Answer from the drawing. Dimensions are ordinates in mm from the lowest x, y and z of the part. Coordinates: 2 decimals unless noted, no trailing zeros. Order: outer loops, then holes, each group sorted by start corner. A loop starts at its lowest first (then second) coordinate and runs counter-clockwise, first axis right, second up.
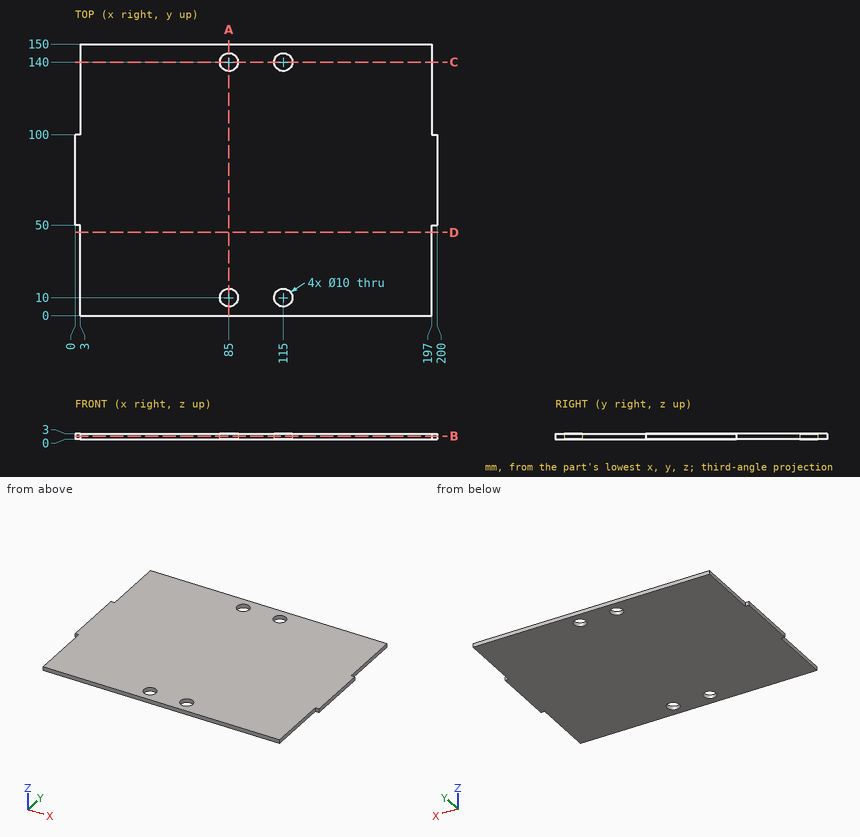
1. The part is cut by section B-B (z = 1.6). Determine the outline of the cut face in (x, y), plus the area to 3 significant figures.
2. Consider probe 1 along Y at (x, z) = (85, 1.95); probe 2 along Y at (x, z) = (84, 2.1); probe 3 along X at (y, z) = (144.5, 0.7). Determine where each line is inside the solid, lowest interval first.
3. The part is cut by section C-C (y = 140). Determine the outline of the cut face in (x, z).
4. The part is cut by section D-D (y = 46). Determine the outline of the cut face in (x, z), plus the area to 3 significant figures.
5. Flat-ended cylindrical pins translate along their axes: pin 1 (1.5 mm diameter, centred on x = 198, z = 1.5, fed in from +Y); pin 2 (1.5 mm diameter, centred on y = 107, z = 0.5, fed in from -X); pin 3 (1.5 mm diameter, centred on x = 1.5, z = 1.5, fed in from -Y). Find the tip coordinate at first contact, or state that the pin passes through.
6. The part is cut by section A-A (x = 85). Determine the outline of the cut face in (y, z).
Worked out:
1. outline: (0, 50) - (3, 50) - (3, 0) - (197, 0) - (197, 50) - (200, 50) - (200, 100) - (197, 100) - (197, 150) - (3, 150) - (3, 100) - (0, 100) - close; hole circle Ø10 at (85, 10); hole circle Ø10 at (85, 140); hole circle Ø10 at (115, 10); hole circle Ø10 at (115, 140)
1. area: 29,100 mm2
2. probe 1: y = 0 to 5, 15 to 135, 145 to 150
2. probe 2: y = 0 to 5.1, 14.9 to 135.1, 144.9 to 150
2. probe 3: x = 3 to 82.82, 87.18 to 112.82, 117.18 to 197
3. outline: (3, 0) - (80, 0) - (80, 3) - (3, 3) - close; (90, 0) - (110, 0) - (110, 3) - (90, 3) - close; (120, 0) - (197, 0) - (197, 3) - (120, 3) - close
4. outline: (3, 0) - (197, 0) - (197, 3) - (3, 3) - close
4. area: 582 mm2
5. pin 1: stops at y = 100
5. pin 2: stops at x = 3
5. pin 3: stops at y = 50
6. outline: (0, 0) - (5, 0) - (5, 3) - (0, 3) - close; (15, 0) - (135, 0) - (135, 3) - (15, 3) - close; (145, 0) - (150, 0) - (150, 3) - (145, 3) - close
